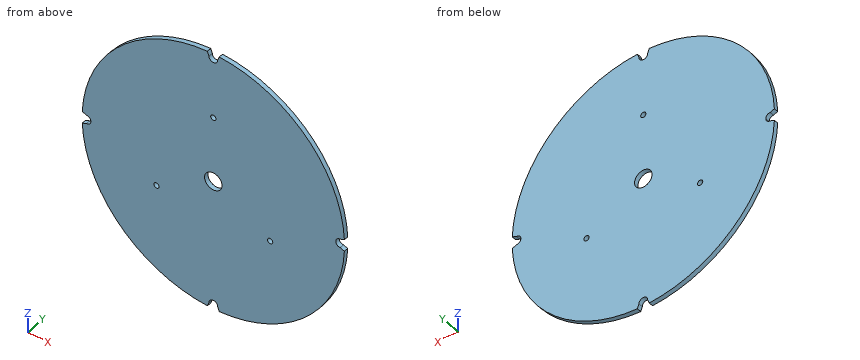
```python
from build123d import *

# Parameters (mm, degrees)
SKETCH1_R               = 10
BOSS_EXTRUDE1_DEPTH     = 5
CUT_EXTRUDE1_DEPTH      = 212.975206598
CUT_EXTRUDE1_DEPTH_BACK = 212.975206598
SKETCH2_R               = 3


with BuildPart() as part:
    # Sketch1 → Boss-Extrude1 (new body)
    with BuildSketch(Plane(origin=(0, 0, 0), x_dir=(1, 0, 0), z_dir=(0, 1, 0))):
        with BuildLine():
            ThreePointArc((5, 145), (0, 140), (-5, 145))
            Line((-5, 145), (-6.764310309, 149.847402734))
            ThreePointArc((-6.764310309, 149.847402734), (-106.066017178, 106.066017178), (-149.847402734, 6.764310309))
            Line((-149.847402734, 6.764310309), (-145, 5))
            ThreePointArc((-145, 5), (-141.464466094, 3.535533906), (-140, 0))
            ThreePointArc((-140, 0), (-141.464466094, -3.535533906), (-145, -5))
            Line((-145, -5), (-149.847402734, -6.764310309))
            ThreePointArc((-149.847402734, -6.764310309), (-106.066017178, -106.066017178), (-6.764310309, -149.847402734))
            Line((-6.764310309, -149.847402734), (-5, -145))
            ThreePointArc((-5, -145), (0, -140), (5, -145))
            Line((5, -145), (6.764310309, -149.847402734))
            ThreePointArc((6.764310309, -149.847402734), (106.066017178, -106.066017178), (149.847402734, -6.764310309))
            Line((149.847402734, -6.764310309), (145, -5))
            ThreePointArc((145, -5), (140, 0), (145, 5))
            Line((145, 5), (149.847402734, 6.764310309))
            ThreePointArc((149.847402734, 6.764310309), (106.066017178, 106.066017178), (6.764310309, 149.847402734))
            Line((6.764310309, 149.847402734), (5, 145))
        make_face()
        with Locations(Location((0, 0, 0), (0, 0, 270))):
            Circle(SKETCH1_R, mode=Mode.SUBTRACT)
    extrude(amount=BOSS_EXTRUDE1_DEPTH)

    # Sketch2 → Cut-Extrude1 (cut, two sides: drawn at the far end of the back side and taken through both)
    with BuildSketch(Plane(origin=(0, 5, 0), x_dir=(1, 0, 0), z_dir=(0, 1, 0)).offset(-CUT_EXTRUDE1_DEPTH_BACK)):
        with Locations(Location((0, -75, 0), (0, 0, 270))):
            Circle(SKETCH2_R)
        with Locations(Location((64.951905284, 37.5, 0), (0, 0, 270))):
            Circle(SKETCH2_R)
        with Locations(Location((-64.951905284, 37.5, 0), (0, 0, 270))):
            Circle(SKETCH2_R)
    extrude(amount=CUT_EXTRUDE1_DEPTH + CUT_EXTRUDE1_DEPTH_BACK, mode=Mode.SUBTRACT)


solid = part.part
```
Source: CAD feature listing. Evaluate the final solid. Frame: model axes, mm. Coordinates: 2 decimals unless noted, no trailing zeros. Write each loop counter-clockwise with the first axis right and the second up, starting at its lowest first coordinate (ties: lowest second). Pieces come first, ordered by that corner, then holes. Notation, with made-up numbers: M -31.5,-15 L -21.5,-15 A15 cw -21.5,-9 Z; hole C 74.25,50 d11. An arc over 180 degrees is marked long. Answer as a JSON object with one key per item and string values.
1. Cut plane A-A on y = 2.5. Output: boundary loops of the cut face in (x, z).
Evaluation:
{"outline": "M -149.85,-6.76 A150 ccw -6.76,-149.85 L -5,-145 A5 cw 5,-145 L 6.76,-149.85 A150 ccw 149.85,-6.76 L 145,-5 A5 cw 145,5 L 149.85,6.76 A150 ccw 6.76,149.85 L 5,145 A5 cw -5,145 L -6.76,149.85 A150 ccw -149.85,6.76 L -145,5 A5 cw -145,-5 Z; hole C -64.95,-37.5 d6; hole C 0,0 d20; hole C 0,75 d6; hole C 64.95,-37.5 d6"}
2. Cut plane B-B on z = -65. Output: boundary loops of the cut face in (x, y), plus the area to 3 significant figures.
Evaluation:
{"outline": "M -135.19,0 L 135.19,0 L 135.19,5 L -135.19,5 Z", "area": "1,350 mm^2"}
3. Contact query for flat-ended pins moving along their axis: P1, Ø5.5, axis at x = 64.95, z = -37.5, coming from the +Y side; P2, Ø1, axis at x = 15.5, y = 0.5, coming from the +Z side; P3, Ø2, axis at y = 2.5, z = -69.5, coming from the -X side; P4, Ø1, axis at y = 2.5, z = 83.5, coming from the -X side. Output: stop coordinate, or through.
Evaluation:
{"P1": "through", "P2": "z = 149.25", "P3": "x = -133.45", "P4": "x = -124.94"}
4. Cut plane C-C on z = 33. Output: boundary loops of the cut face in (x, y).
Evaluation:
{"outline": "M -146.32,0 L 146.32,0 L 146.32,5 L -146.32,5 Z"}
5. Ray query, L1, parallel to X at y = 2.55, z = 0; L2, parallel to X at y = 1.05, z = -37.5; L3, parallel to X at y = 3.95, z = 1.5. Return the intervals inside material, ascending.
Evaluation:
{"L1": "-140 to -10, 10 to 140", "L2": "-145.24 to -67.95, -61.95 to 61.95, 67.95 to 145.24", "L3": "-140.23 to -9.89, 9.89 to 140.23"}
